Input: part model. Units: mm. Frame: model coordinates. Face numbers are marked on the shaded views. A direction names the side the tool comes from. Coordinates: 2 decimals unless noted, no trailing zeros. Order: outer loops, then holes, each group sorted by start corner. A loop starts at its lowest first (then second) coordinate and runs counter-clockwise, first axis right, second up. Notation, with made-up numbers: (-22.5, -20.75) - (-18.5, -20.75) arc R28 cw to (-18.5, 13.25) - close; hole circle Ø11 at (-38, 30). An arc over 180 degrees is marked (long way). Answer as CSV lines item,"result". Start each with the question number.
Item 1: Material intervals for line 1 along X through (y, z) = (0, -9.5); line 2 along Z through (x, y) = (0.7, 2.3), sorted ascending.
Item 2: Draft query along Y for the marked faces 1 and 2. Return one class per face: +Y half, -Y half, draft (parallel to the pull), parting line (faces both ways), or undercut.
Item 3: Section D-D (z = -21.75). Output: boundary loops of the cut face in (x, y), and give its area (3 significant figures).
Item 4: First-contact query: pin 1 (1.5 mm diameter, centred on x = -1.5, z = -13.5, fed in from -Y); pin 2 (3 mm diameter, centred on y = -1, z = -21.5, fed in from -X). Flat tips, straight axial feed; report the tip coordinate or a pass-through.
Item 5: Access query for the marked faces 3 and 4. Directions: +Z, -Z, +X, -X, +Y, -Y. A direction counts if a zero-diameter tool reaches every point of the face in a straight line with its end or side. Return the directions, or none.
Item 6: Section C-C (z = -15). Output: boundary loops of the cut face in (x, y).
Item 7: Section A-A (x = 0). Output: boundary loops of the cut face in (y, z), and give its area (3 significant figures).
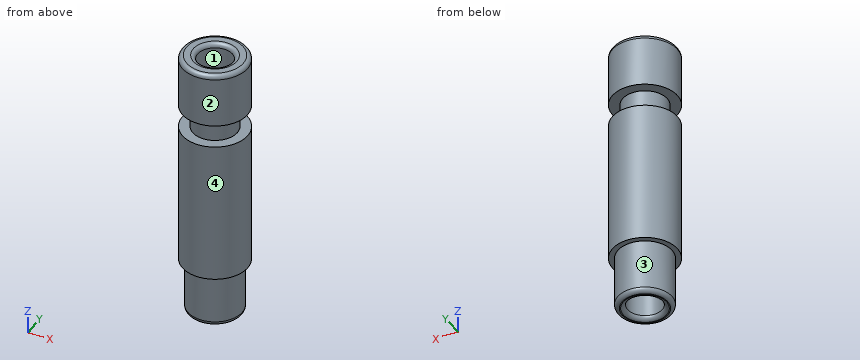
Autodesk Inventor part; units mm, degrees
ref_plane "YZ Plane" through (0, 0, 0) normal (1, 0, 0) x (0, 1, 0)
ref_plane "XZ Plane" through (0, 0, 0) normal (0, 1, 0) x (-1, 0, 0)
ref_plane "XY Plane" through (0, 0, 0) normal (0, 0, 1) x (1, 0, 0)
sketch "Эскиз1" plane through (0, 0, 0) normal (0, 1, 0) x (-1, 0, 0)
  line L0 (0, 0) -> (0, -25.3) construction
  line L1 (0, 0) -> (-3, 0) construction
  line L2 (-3, 0) -> (-3, -5)
  line L3 (0, -5) -> (-2.05, -5) construction
  line L4 (-2.05, -5) -> (-2.05, -7.1)
  line L5 (-3, -5) -> (-2.05, -5)
  line L6 (-2.05, -7.1) -> (-3, -7.1)
  line L7 (0, 0) -> (-1.6, 0) construction
  line L8 (-1.6, 0) -> (-3, 0) construction
  line L9 (-1.6, 0) -> (-3, 0)
  line L10 (-1.6, 0) -> (-1.6, -25.3)
  line L11 (0, -25.3) -> (-2.5, -25.3) construction
  line L12 (-1.6, -25.3) -> (-2.5, -25.3)
  line L13 (-2.5, -25.3) -> (-2.5, -20.3)
  line L14 (-2.5, -20.3) -> (-3, -20.3)
  line L15 (-3, -20.3) -> (-3, -7.1)
  dimension "d4" = 25.3
  dimension "d5" = 3
  dimension "d6" = 5
  dimension "d7" = 2.05
  dimension "d8" = 2.1
  dimension "d9" = 1.6
  dimension "d10" = 25.3
  dimension "d11" = 2.5
  dimension "d12" = 5
revolve "Вращение1" add sketch "Эскиз1" angle 360 about axis through (0, 0, 0) along (0, 0, -1)
fillet "Сопряжение1" radius 0.4 4 edges at (-2.5, 0, -25.3) (-3, 0, 0) (-1.6, 0, 0) (-1.6, 0, -25.3)
thread "Резьба1"
thread "Резьба2"
properties part number "BREAK"
Determined:
1,line 1,"x = -3 to -1.6, 1.6 to 3"
1,line 2,"z = -25.16 to -7.1, -5 to 0"
2,face 1,"undercut"
2,face 2,"parting line"
3,outline,"circle Ø5 at (0, 0); hole circle Ø3.2 at (0, 0)"
3,area,"11.6 mm^2"
4,pin 1,"stops at y = -2.9"
4,pin 2,"stops at x = -3"
5,face 3,"-Z"
5,face 4,"+Z, -Z"
6,outline,"circle Ø6 at (0, 0); hole circle Ø3.2 at (0, 0)"
7,outline,"(-3, -20.3) - (-2.5, -20.3) - (-2.5, -24.9) arc R0.4 ccw to (-2.1, -25.3) - (-2, -25.3) arc R0.4 ccw to (-1.6, -24.9) - (-1.6, -0.4) arc R0.4 ccw to (-2, 0) - (-2.6, 0) arc R0.4 ccw to (-3, -0.4) - (-3, -5) - (-2.05, -5) - (-2.05, -7.1) - (-3, -7.1) - close; (1.6, -24.9) arc R0.4 ccw to (2, -25.3) - (2.1, -25.3) arc R0.4 ccw to (2.5, -24.9) - (2.5, -20.3) - (3, -20.3) - (3, -7.1) - (2.05, -7.1) - (2.05, -5) - (3, -5) - (3, -0.4) arc R0.4 ccw to (2.6, 0) - (2, 0) arc R0.4 ccw to (1.6, -0.4) - close"
7,area,"61.6 mm^2"
